from build123d import *

# Parameters (mm, degrees)
EXTRUDE_THIN1_DEPTH = 6


with BuildPart() as part:
    # Sketch2 → Extrude-Thin1 (new body)
    with BuildSketch(Plane.XY):
        with BuildLine():
            Line((189.55, -6.1), (0, -6.1))
            ThreePointArc((0, -6.1), (-6.1, 0), (0, 6.1))
            Line((0, 6.1), (189.55, 6.1))
            Line((189.55, 6.1), (189.55, 7.1))
            Line((189.55, 7.1), (0, 7.1))
            ThreePointArc((0, 7.1), (-7.1, 0), (0, -7.1))
            Line((0, -7.1), (189.55, -7.1))
            Line((189.55, -7.1), (189.55, -6.1))
        make_face()
    extrude_thin1 = extrude(amount=EXTRUDE_THIN1_DEPTH)

    # Mirror1: Extrude-Thin1 across plane
    add(extrude_thin1.mirror(Plane(origin=(189.55, 7.1, 6), x_dir=(0, 0, 1), z_dir=(1, 0, 0))))


solid = part.part
Part model, mm, in its own coordinate system. A direction names the side the tool comes from. Round coordinates to 2 decimals unless told otherwise and drop trailing zeros. Loops run counter-clockwise (first coordinate to the right, second up) from the corner with the lowest first, then second, coordinate; pieces in that order, holes last. Notation, with made-up numbers: (77, 78) - (95, 78) arc R21 ccw to (95, 101) - close; hole circle Ø4 at (35, 81). An arc over 180 degrees is marked (long way). Answer as a JSON object with one key per item and string values.
Item 1: Band-saw the part on C-C on y = -2.5. List the corners of the cut face in (x, z), plus the area to 3 significant figures.
Output:
{"outline": "(-6.65, 0) - (-5.56, 0) - (-5.56, 6) - (-6.65, 6) - close; (384.66, 0) - (385.75, 0) - (385.75, 6) - (384.66, 6) - close", "area": "13.0 mm2"}
Item 2: Pull direction Y, two halves, no side cores. Call faces 3 (the face through (385.2, -0.1, 3)), 4 (the face through (190.5, 6.3, 6)), 5 (the face through (192, -7.1, 3)): pulls with the +Y half, pulls with the -Y half, needs draft (parallel to the pull), parting line crosses it, or undercut.
Output:
{"face 3": "undercut", "face 4": "needs draft", "face 5": "pulls with the -Y half"}
Item 3: Wall check: L1, parallel to Y at x = 236.5, z = 5; L2, parallel to X at y = -0.75, z = 3.05; L3, parallel to X at y = 1, z = 1.2. Give the ranges that are in metal, low to high.
Output:
{"L1": "-7.1 to -6.1, 6.1 to 7.1", "L2": "-7.06 to -6.05, 385.15 to 386.16", "L3": "-7.03 to -6.02, 385.12 to 386.13"}
Item 4: Tool access for faces 1 (the face through (192, 6.1, 3)), 2 (the face through (-7.1, 0.16, 2.96)): list every direction of +Z, -Z, +X, -X, +Y, -Y with a clear straight run to the whole face (end or side of a thin tool).
Output:
{"face 1": "+Z, -Z", "face 2": "+Z, -Z, -X"}
Item 5: Pin check, flat tip, straight feed: pin 1 (3 mm diameter, centred on x = 267.5, y = 4.5, fed in from -Z). Stop position of the tip, or through.
Output:
{"pin 1": "through"}
Item 6: Band-saw the part on B-B on z = 4.55. List the corners of the cut face in (x, y).
Output:
{"outline": "(0, -7.1) - (379.1, -7.1) arc R7.1 ccw to (379.1, 7.1) - (0, 7.1) arc R7.1 ccw to start; hole (0, -6.1) - (379.1, -6.1) arc R6.1 ccw to (379.1, 6.1) - (0, 6.1) arc R6.1 ccw to start"}
Item 7: Band-saw the part on A-A on x = 130. List the corners of the cut face in (y, z).
Output:
{"outline": "(-7.1, 0) - (-6.1, 0) - (-6.1, 6) - (-7.1, 6) - close; (6.1, 0) - (7.1, 0) - (7.1, 6) - (6.1, 6) - close"}
